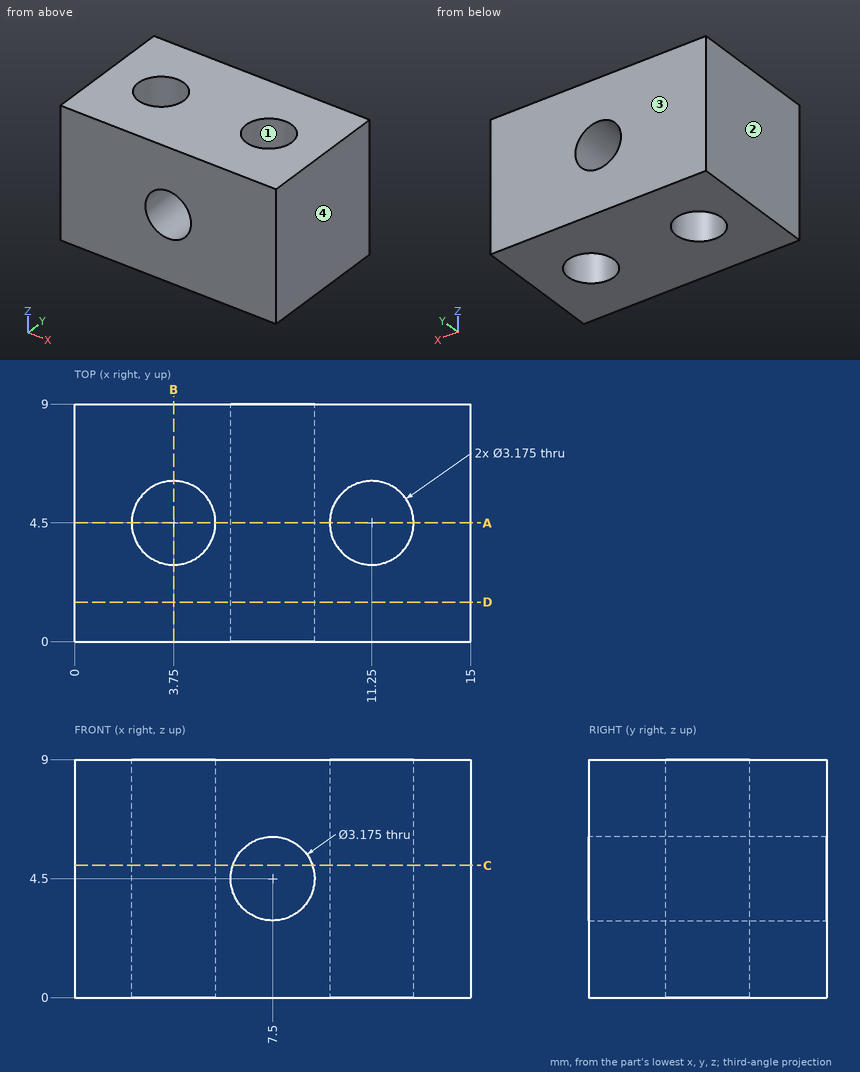
Check sheet for the drawn part. Datum: minimum x, y, z corner. Units: mm. Round coordinates to 2 decimals unless told otherwise and drop trailing zeros. Loops run counter-clockwise (first coordinate to the right, second up) from the corner with the lowest first, then second, coordinate; pieces in that order, holes last.
Item 1: Cross-section at C-C on z = 5. Count the separate pieces of the cut face and the enclosed holes in it, then the cut area to 3 significant figures.
Item 2: Mould release check, pull along X, two halves, no side actions. Record for the marked faces 1, 2, 3 and 4: pulls with the +X half, pulls with the -X half, needs draft (parallel to the pull), parting line crosses it, or undercut.
Item 3: Cross-section at B-B on x = 3.75. Record the boundary of the cut face in (y, z), then the cut area to 3 significant figures.
Item 4: Gauge pin test, flat end, axial feed: pin 1 (3 mm diameter, centred on x = 2, y = 5, fed in from -Z). Record the tip position at first contact, or that the pin passes through.
Item 5: Cross-section at D-D on y = 1.5. Record the boundary of the cut face in (x, z) (1 decimal).
Item 6: Thickness scan on line 1 (X direction, y = 7, z = 4.5); line 2 (X direction, y = 3.5, z = 7.5); line 3 (Y direction, x = 11.25, z = 4.5). Record the ranges inside material, lowest first.
Item 7: Cross-section at A-A on y = 4.5. Record the boundary of the cut face in (x, z) (1 decimal), then the cut area to 3 significant figures.
Answer sheet:
1. separate pieces: 2
1. enclosed holes: 2
1. area: 92.0 mm2
2. face 1: undercut
2. face 2: pulls with the -X half
2. face 3: needs draft
2. face 4: pulls with the +X half
3. outline: (0, 0) - (2.91, 0) - (2.91, 9) - (0, 9) - close; (6.09, 0) - (9, 0) - (9, 9) - (6.09, 9) - close
3. area: 52.4 mm2
4. pin 1: stops at z = 0
5. outline: (0, 0) - (15, 0) - (15, 9) - (0, 9) - close; hole circle Ø3.2 at (7.5, 4.5)
6. line 1: x = 0 to 5.91, 9.09 to 15
6. line 2: x = 0 to 2.52, 4.98 to 10.02, 12.48 to 15
6. line 3: y = 0 to 2.91, 6.09 to 9
7. outline: (0, 0) - (2.2, 0) - (2.2, 9) - (0, 9) - close; (5.3, 0) - (9.7, 0) - (9.7, 9) - (5.3, 9) - close; (12.8, 0) - (15, 0) - (15, 9) - (12.8, 9) - close; hole circle Ø3.2 at (7.5, 4.5)
7. area: 69.9 mm2
